Can you work these out from the model? Positions are in its coordinate system, mm. A direction names the side the tool comes from. Coordinates: 2 decimals unless noted, no trailing zeros. Order: outer loops, then holes, each group sorted by start corner. A loop starts at its lowest first (then second) coordinate and runs counter-clockwise, first axis right, second up. Notation, with made-up numbers: M 3,52.5 L 26,52.5 A10 cw 26,67.5 Z; hole C -27,26 d6. An arc over 180 degrees is marked long. Answer as a JSON object with one key per item and string values.
from build123d import *

# Parameters (mm, degrees)
SKETCH1_W            = 13
SKETCH1_H            = 15
BOSS_EXTRUDE1_DEPTH  = 150
SKETCH5_R            = 2.5
CUT_EXTRUDE3_DEPTH   = 151.748963512
SKETCH8_W            = 13
SKETCH8_H            = 15
BOSS_EXTRUDE3_DEPTH  = 15
SKETCH10_R           = 1.6
CUT_EXTRUDE4_DEPTH   = 151.888203648
SKETCH11_W           = 30
SKETCH11_H           = 30
BOSS_EXTRUDE4_DEPTH  = 13
SKETCH12_R           = 2.5
CUT_EXTRUDE5_DEPTH   = 152.307633647
FILLET1_R            = 5
FILLET2_R            = 5
SKETCH13_R           = 3
CUT_EXTRUDE6_DEPTH   = 152.81732444
SKETCH15_W           = 13
SKETCH15_H           = 15
BOSS_EXTRUDE5_DEPTH  = 40
SKETCH23_W           = 10
SKETCH23_H           = 15
BOSS_EXTRUDE10_DEPTH = 54.49
SKETCH24_W           = 10
SKETCH24_H           = 15
BOSS_EXTRUDE11_DEPTH = 54.49
SKETCH27_W           = 10
SKETCH27_H           = 10
BOSS_EXTRUDE13_DEPTH = 50
SKETCH28_W           = 90
SKETCH28_H           = 13
CUT_EXTRUDE15_DEPTH  = 175.48432623
CHAMFER1_SIZE        = 10
FILLET3_R            = 5


with BuildPart() as part:
    # Sketch1 → Boss-Extrude1 (new body)
    with BuildSketch(Plane(origin=(0, 0, 0), x_dir=(0, 0, -1), z_dir=(1, 0, 0))):
        Rectangle(SKETCH1_W, SKETCH1_H)
    extrude(amount=BOSS_EXTRUDE1_DEPTH)

    # Sketch5 → Cut-Extrude3 (cut, through all)
    with BuildSketch(Plane.XY.offset(6.5)):
        with Locations((115, 0)):
            Circle(SKETCH5_R)
        with Locations((125, 0)):
            Circle(SKETCH5_R)
        with Locations((105, 0)):
            Circle(SKETCH5_R)
    extrude(amount=-CUT_EXTRUDE3_DEPTH, mode=Mode.SUBTRACT)

    # Sketch8 → Boss-Extrude3 (add)
    with BuildSketch(Plane.ZY):
        Rectangle(SKETCH8_W, SKETCH8_H)
    extrude(amount=BOSS_EXTRUDE3_DEPTH)

    # Sketch10 → Cut-Extrude4 (cut, through all)
    with BuildSketch(Plane(origin=(0, -7.5, 0), x_dir=(-1, 0, 0), z_dir=(0, -1, 0))):
        with Locations(Location((7, 0, 0), (0, 0, 90))):
            Circle(SKETCH10_R)
        with Locations(Location((-12, 0, 0), (0, 0, 90))):
            Circle(SKETCH10_R)
    extrude(amount=-CUT_EXTRUDE4_DEPTH, mode=Mode.SUBTRACT)

    # Sketch11 → Boss-Extrude4 (add)
    with BuildSketch(Plane(origin=(0, 0, -6.5), x_dir=(-1, 0, 0), z_dir=(0, 0, -1))):
        with Locations((-115, 0)):
            Rectangle(SKETCH11_W, SKETCH11_H)
    extrude(amount=-BOSS_EXTRUDE4_DEPTH)

    # Sketch12 → Cut-Extrude5 (cut, through all)
    with BuildSketch(Plane(origin=(0, 0, -6.5), x_dir=(-1, 0, 0), z_dir=(0, 0, -1))):
        with Locations((-115, 10)):
            Circle(SKETCH12_R)
        with Locations((-105, 0)):
            Circle(SKETCH12_R)
        with Locations((-125, 0)):
            Circle(SKETCH12_R)
        with Locations((-115, 0)):
            Circle(SKETCH12_R)
        with Locations((-115, -10)):
            Circle(SKETCH12_R)
    extrude(amount=-CUT_EXTRUDE5_DEPTH, mode=Mode.SUBTRACT)

    # Fillet1
    fillet1_edges = [part.edges().sort_by_distance(p)[0] for p in [
        (100, 15, 0),
        (130, -15, 0),
        (100, -15, 0),
        (130, 15, 0),
    ]]
    fillet(fillet1_edges, radius=FILLET1_R)

    # Fillet2
    fillet2_edges = [part.edges().sort_by_distance(p)[0] for p in [
        (150, -7.5, 0),
        (150, 7.5, 0),
    ]]
    fillet(fillet2_edges, radius=FILLET2_R)

    # Sketch13 → Cut-Extrude6 (cut, through all)
    with BuildSketch(Plane(origin=(0, 7.5, 0), x_dir=(1, 0, 0), z_dir=(0, 1, 0))):
        with Locations(Location((2.5, 0, 0), (0, 0, 270))):
            Circle(SKETCH13_R)
    extrude(amount=-CUT_EXTRUDE6_DEPTH, mode=Mode.SUBTRACT)

    # Sketch15 → Boss-Extrude5 (add)
    with BuildSketch(Plane.ZY.offset(15)):
        Rectangle(SKETCH15_W, SKETCH15_H)
    extrude(amount=BOSS_EXTRUDE5_DEPTH)

    # Sketch23 → Boss-Extrude10 (add)
    with BuildSketch(Plane.XY.offset(6.5)):
        with Locations((40, 0)):
            Rectangle(SKETCH23_W, SKETCH23_H)
    extrude(amount=BOSS_EXTRUDE10_DEPTH)

    # Sketch24 → Boss-Extrude11 (add)
    with BuildSketch(Plane(origin=(0, 0, -6.5), x_dir=(-1, 0, 0), z_dir=(0, 0, -1))):
        with Locations((-40, 0)):
            Rectangle(SKETCH24_W, SKETCH24_H)
    extrude(amount=BOSS_EXTRUDE11_DEPTH)

    # Sketch27 → Boss-Extrude13 (add)
    with BuildSketch(Plane(origin=(0, 7.5, 0), x_dir=(1, 0, 0), z_dir=(0, 1, 0))):
        with Locations((40, 55.99)):
            Rectangle(SKETCH27_W, SKETCH27_H)
        with Locations((40, -55.99)):
            Rectangle(SKETCH27_W, SKETCH27_H)
    extrude(amount=BOSS_EXTRUDE13_DEPTH)

    # Sketch28 → Cut-Extrude15 (cut, through all)
    with BuildSketch(Plane.XZ.offset(7.5)):
        with Locations((-10, 0)):
            Rectangle(SKETCH28_W, SKETCH28_H)
    extrude(amount=-CUT_EXTRUDE15_DEPTH, mode=Mode.SUBTRACT)

    # Chamfer1
    chamfer1_edges = [part.edges().sort_by_distance(p)[0] for p in [
        (40, 7.5, -50.99),
        (40, 7.5, 50.99),
    ]]
    chamfer(chamfer1_edges, length=CHAMFER1_SIZE)

    # Fillet3
    fillet3_edges = [part.edges().sort_by_distance(p)[0] for p in [
        (40, -7.5, 60.99),
        (40, -7.5, -60.99),
    ]]
    fillet(fillet3_edges, radius=FILLET3_R)


solid = part.part
Item 1: Which directions (+Z, -Z, +X, -X, +Y, -Y) give clear straight access to the entire face, cutting with the end or side of a thin tool? Please do faces 4 (the flat face through (45, 10, -45)), 5 (the flat face through (45, 10, 45)), 6 (the flat face through (51, -7.5, 0)).
Answers follow:
{"face 4": "-Z, +X, +Y, -Y", "face 5": "+Z, +X, +Y, -Y", "face 6": "+Z, -Z, -X, -Y"}
Item 2: Please list where these lines run through material, in increasing order: line 1 (Y direction, x = 115, z = -1); line 2 (Y direction, x = 125, z = 0); line 3 (Z direction, x = 101, y = 1).
Answers follow:
{"line 1": "y = -15 to -12.5, -7.5 to -2.5, 2.5 to 7.5, 12.5 to 15", "line 2": "y = -15 to -2.5, 2.5 to 15", "line 3": "z = -6.5 to 6.5"}
Item 3: I'm going to push flat-ended pins straight in: pin 1 (4.5 mm diameter, centred on x = 105, y = 0, fed in from +Z); pin 2 (0.8 mm diameter, centred on y = -9.5, z = -2.5, fed in from -X); pin 3 (6.5 mm diameter, centred on x = 115, y = 0, fed in from +Z); pin 4 (6.5 mm diameter, centred on x = 125, y = 0, fed in from -Z). Where does each tip first touch, or does it pass through?
Answers follow:
{"pin 1": "passes through", "pin 2": "stops at x = 100", "pin 3": "stops at z = 6.5", "pin 4": "stops at z = -6.5"}
Item 4: I want a section at A-A, the plane y = 52. Write out the boundary of the cut face in (x, z), plus the area to 3 significant figures.
Answers follow:
{"outline": "M 35,-60.99 L 45,-60.99 L 45,-50.99 L 35,-50.99 Z; M 35,50.99 L 45,50.99 L 45,60.99 L 35,60.99 Z", "area": "200 mm^2"}
Item 5: I want a section at B-B, the plane x = 115. Write out the boundary of the cut face in (y, z), plus the area to 3 significant figures.
Answers follow:
{"outline": "M -15,-6.5 L -12.5,-6.5 L -12.5,6.5 L -15,6.5 Z; M -7.5,-6.5 L -2.5,-6.5 L -2.5,6.5 L -7.5,6.5 Z; M 2.5,-6.5 L 7.5,-6.5 L 7.5,6.5 L 2.5,6.5 Z; M 12.5,-6.5 L 15,-6.5 L 15,6.5 L 12.5,6.5 Z", "area": "195 mm^2"}
Item 6: I want a section at D-D, the plane y = -4.5. Write out the boundary of the cut face in (x, z).
Answers follow:
{"outline": "M 35,-60.57 L 45,-60.57 L 45,-6.5 L 149.58,-6.5 L 149.58,6.5 L 45,6.5 L 45,60.57 L 35,60.57 Z"}
Item 7: I want a section at C-C, the plane z = -32.5. Write out the boundary of the cut face in (x, y).
Answers follow:
{"outline": "M 35,-7.5 L 45,-7.5 L 45,7.5 L 35,7.5 Z"}
Item 8: If we mould it in two halves opening along Z, with no side actions, what happens to faces 1 (the flat face through (98, 0, -6.5)), 2 (the flat face through (39.93, 12.57, -46.06)), 3 (the cylindrical face through (102.615, 0.751, -0.091))? For each: pulls with the +Z half, pulls with the -Z half, needs draft (parallel to the pull), parting line crosses it, or undercut.
Answers follow:
{"face 1": "pulls with the -Z half", "face 2": "undercut", "face 3": "needs draft"}
